from build123d import *

# Parameters (mm, degrees)
F0_W     = 450
F0_H     = 100
F1_DEPTH = 10
F2_R     = 10
F3_DEPTH = 20.001


# Not quite as in the source:
# - a pattern or mirror of a feature is missing from the dataset's text; its kind, count and spacing are read off the source's solid


with BuildPart() as f1:
    # F0 (on Front) → F1 (new body, symmetric)
    with BuildSketch(Plane.XZ):
        Rectangle(F0_W, F0_H)
    extrude(amount=F1_DEPTH, both=True)

    # F2 (on face) → F3 (cut, through all)
    with BuildSketch(Plane.XZ.offset(10)):
        with Locations((-200, 0)):
            Circle(F2_R)
    f3 = extrude(amount=-F3_DEPTH, mode=Mode.SUBTRACT)

    # F3_copies: F3 across plane
    add(f3.mirror(Plane(origin=(0, 0, 0), x_dir=(0, 0, 1), z_dir=(1, 0, 0))), mode=Mode.SUBTRACT)


solid = f1.part
The model under review builds one solid part; all positions refer to its coordinate system, in mm. Coordinates: 2 decimals unless noted, no trailing zeros. Loops run counter-clockwise (first coordinate to the right, second up) from the corner with the lowest first, then second, coordinate; pieces in that order, holes last. Notation, with made-up numbers: M 63,87 L 109,87 A26 ccw 109,113 Z; hole C 19.25,-17 d5. An arc over 180 degrees is marked long. Put each result on its own line as item: value. Start each with the question number.
Q1. Clearance check with flat-ended pins moving along their axes: pin 1 (23 mm diameter, centred on x = -200, z = 0, fed in from -Y); pin 2 (18 mm diameter, centred on x = 200, z = 0, fed in from -Y). State where each tip first meets the part, or that it passes through.
Q2. Add section B-B (x = -200). Write out the cut boundary in (y, z), and give its area (3 significant figures).
Q3. The part is to be moulded in two halves that separate along Z. For faces 1 (the flat face through (-3, 0, 50)), 2 (the flat face through (-3, 0, -50)), 3 (the cylindrical face through (-190.763, -0.14, -3.83)), 4 (the flat face through (-225, 0, -1)), say which applies: +Z half, -Z half, draft (parallel to the pull), parting line (faces both ways), or undercut.
Q4. Add section A-A (z = 0). Write out the cut boundary in (x, y).
Q5. Wall thickness on line 1 (Z direction, x = 200, y = -1.25); line 2 (X direction, y = 3, z = 7): over which ranges is each line inside the solid? List them lowest first.
Answers:
1. pin 1: stops at y = -10
1. pin 2: passes through
2. outline: M -10,-50 L 10,-50 L 10,-10 L -10,-10 Z; M -10,10 L 10,10 L 10,50 L -10,50 Z
2. area: 1,600 mm^2
3. face 1: +Z half
3. face 2: -Z half
3. face 3: undercut
3. face 4: draft
4. outline: M -225,-10 L -210,-10 L -210,10 L -225,10 Z; M -190,-10 L 190,-10 L 190,10 L -190,10 Z; M 210,-10 L 225,-10 L 225,10 L 210,10 Z
5. line 1: z = -50 to -10, 10 to 50
5. line 2: x = -225 to -207.14, -192.86 to 192.86, 207.14 to 225
